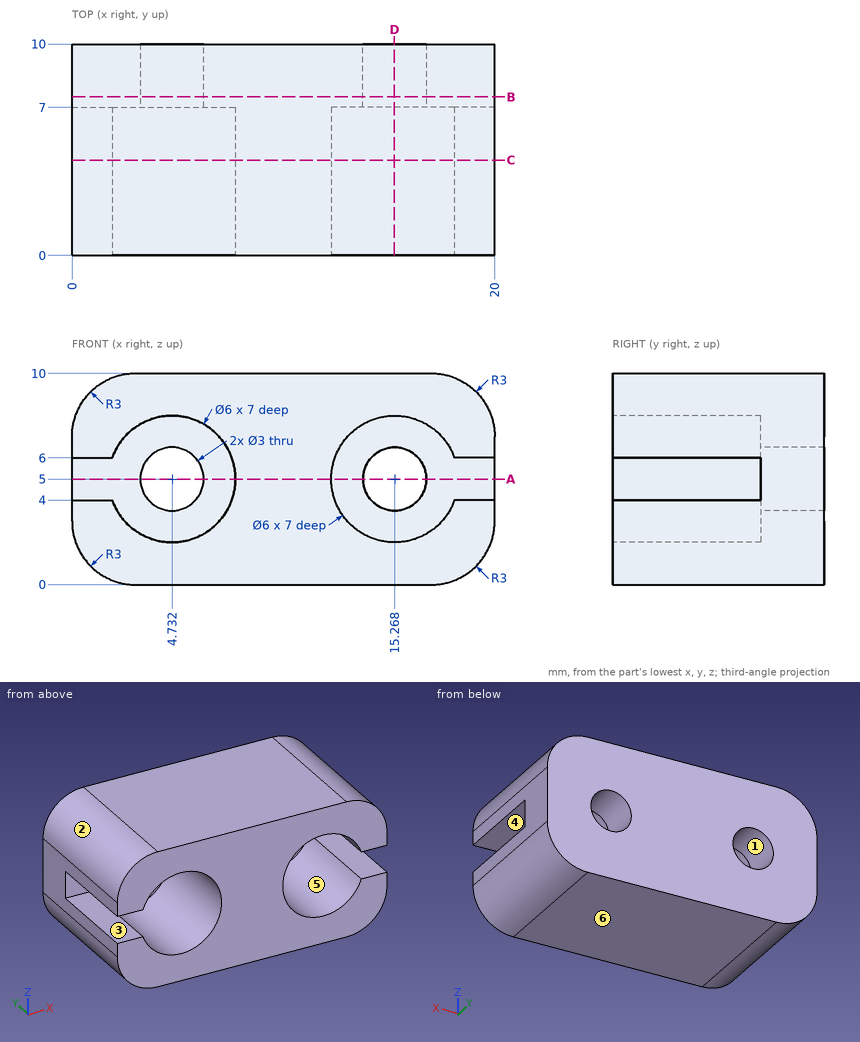
Drawing for the job (mm, zero at the part's lowest x, y, z). A direction names the side the tool comes from. Coordinates: 2 decimals unless noted, no trailing zeros. Write each loop counter-clockwise with the first axis right and the second up, starting at its lowest first coordinate (ties: lowest second). Pieces come first, ordered by that corner, then holes. Notation, with made-up numbers: (-32.75, 47.25) - (-22.75, 47.25) arc R16 cw to (-22.75, 64.25) - close; hole circle Ø6 at (10, -22.5). An arc over 180 degrees is marked (long way). Write each question's results on one line, items separated by ' | '. Start each with the question number.
1) Cut at A-A (z = 5). Write the cut outline in (x, y).
2) Probe line 1 along X through (y, z) = (1.5, 6.5); line 2 along X through (y, z) = (8, 4.5); line 3 along Y through (x, z) = (6.5, 6.25). List the from-to ranges inside material, lowest first. Write a range as from..to.
3) 3-axis set-ups, long thin cutter, end or side, ignore diameter. For the marked faces 4, 5 and 6: which of +Z, -Z, +X, -X, +Y, -Y reach the whole face in a straight line?
4) Cut at B-B (y = 7.5). Write the cut outline in (x, z), then the cut area to 3 significant figures.
5) Mould opens along X. For the marked faces 1, 2 and 3 say: pulls with the +X half, pulls with the -X half, needs draft (parallel to the pull), parting line crosses it, or undercut.
6) Cut at D-D (x = 15.25). Write the cut outline in (y, z), then the cut area to 3 significant figures.
7) Cut at C-C (y = 4.5). Write the cut outline in (x, z), then the cut area to 3 significant figures.
8) Flat gauge pins, fed straight in: P1, Ø0.6, axis at x = 19, y = 4, coming from the +Z side; P2, Ø1, axis at x = 1.5, y = 4.5, coming from the +Z side; P3, Ø2, axis at x = 1, y = 4.5, coming from the -Z side. Where does each tip first touch, or does it go through?
Returned:
1) outline: (0, 7) - (3.23, 7) - (3.23, 10) - (0, 10) - close; (6.23, 7) - (7.73, 7) - (7.73, 0) - (12.27, 0) - (12.27, 7) - (13.77, 7) - (13.77, 10) - (6.23, 10) - close; (16.77, 7) - (20, 7) - (20, 10) - (16.77, 10) - close
2) line 1: 0..2.13, 7.33..12.67, 17.87..20 | line 2: 0..3.32, 6.15..13.85, 16.68..20 | line 3: 7..10
3) face 4: +X, -Y | face 5: -Y | face 6: -Z, +X, -X, +Y, -Y
4) outline: (0, 3) arc R3 ccw to (3, 0) - (17, 0) arc R3 ccw to (20, 3) - (20, 7) arc R3 ccw to (17, 10) - (3, 10) arc R3 ccw to (0, 7) - close; hole circle Ø3 at (4.73, 5); hole circle Ø3 at (15.27, 5) | area: 178 mm^2
5) face 1: undercut | face 2: pulls with the -X half | face 3: needs draft
6) outline: (0, 0) - (10, 0) - (10, 3.5) - (7, 3.5) - (7, 2) - (0, 2) - close; (0, 8) - (7, 8) - (7, 6.5) - (10, 6.5) - (10, 10) - (0, 10) - close | area: 49.0 mm^2
7) outline: (0, 3) arc R3 ccw to (3, 0) - (17, 0) arc R3 ccw to (20, 3) - (20, 4) - (18.1, 4) arc R3 cw (long way) to (18.1, 6) - (20, 6) - (20, 7) arc R3 ccw to (17, 10) - (3, 10) arc R3 ccw to (0, 7) - (0, 6) - (1.9, 6) arc R3 cw (long way) to (1.9, 4) - (0, 4) - close | area: 129 mm^2
8) P1: z = 9.47 | P2: z = 9.83 | P3: z = 0.17
